```python
from build123d import *

# Parameters (mm, degrees)
SKETCH1_R          = 27.5
SKETCH1_R_2        = 48.5
BASE_EXTRUDE_DEPTH = 10


with BuildPart() as part:
    # Sketch1 → Base-Extrude (new body)
    with BuildSketch(Plane.XY):
        with BuildLine():
            Line((70.930675146, 17.258022001), (31.072409725, 181.075965699))
            ThreePointArc((31.072409725, 181.075965699), (-37.180312094, 232.965036888), (-101.966927205, 176.808076081))
            Line((-101.966927205, 176.808076081), (-104.698317648, 161.317591117))
            ThreePointArc((-104.698317648, 161.317591117), (-124.339394775, 129.702595413), (-160.381803445, 120.416872968))
            ThreePointArc((-160.381803445, 120.416872968), (-227.936557036, 127.643740719), (-295.749262378, 131.804190759))
            ThreePointArc((-295.749262378, 131.804190759), (-329.964920671, 135.496946415), (-363.349263399, 143.853583144))
            Line((-363.349263399, 143.853583144), (-458.454915028, 174.755282581))
            ThreePointArc((-458.454915028, 174.755282581), (-464.263200822, 172.612492824), (-463.535533906, 166.464466094))
            Line((-463.535533906, 166.464466094), (-422.516106966, 125.445039154))
            ThreePointArc((-422.516106966, 125.445039154), (-372.592477248, 89.023301508), (-313.933303895, 69.580741007))
            ThreePointArc((-313.933303895, 69.580741007), (-204.337272048, 38.490168586), (-104.328864588, -16.064687542))
            Line((-104.328864588, -16.064687542), (-41.871079854, -59.798099233))
            ThreePointArc((-41.871079854, -59.798099233), (41.176771055, -60.278300619), (70.930675146, 17.258022001))
        make_face()
        Circle(SKETCH1_R, mode=Mode.SUBTRACT)
        with Locations((-35, 165)):
            Circle(SKETCH1_R_2, mode=Mode.SUBTRACT)
    extrude(amount=BASE_EXTRUDE_DEPTH)


solid = part.part
```
Could you check a few things on this model? Use its own coordinates, in mm. A direction names the side the tool comes from. Coordinates: 2 decimals unless noted, no trailing zeros. Write each loop counter-clockwise with the first axis right and the second up, starting at its lowest first coordinate (ties: lowest second). Pieces come first, ordered by that corner, then holes. Notation, with made-up numbers: (-26, -28) - (7, -28) arc R15 cw to (7, -15) - close; hole circle Ø10 at (8.5, 60.5). An arc over 180 degrees is marked (long way). Use a Markdown table: item, result.
Q1. Imagine slicing it at B-B (z = 1.75). List the corners of the cut face in (x, y) for me, and give its area (3 significant figures).
Geometry check:
| item | result |
|---|---|
| outline | (-463.54, 166.46) - (-422.52, 125.45) arc R200 ccw to (-313.93, 69.58) arc R512 cw to (-104.33, -16.06) - (-41.87, -59.8) arc R73 ccw to (70.93, 17.26) - (31.07, 181.08) arc R68 ccw to (-101.97, 176.81) - (-104.7, 161.32) arc R50 cw to (-160.38, 120.42) arc R1500 ccw to (-295.75, 131.8) arc R250 cw to (-363.35, 143.85) - (-458.45, 174.76) arc R5 ccw to start; hole circle Ø97 at (-35, 165); hole circle Ø55 at (0, 0) |
| area | 59,600 mm2 |
Q2. Imagine slicing it at D-D (y = 138.5). List the corners of the cut face in (x, z) for me.
Geometry check:
| item | result |
|---|---|
| outline | (-435.57, 0) - (-344.35, 0) - (-344.35, 10) - (-435.57, 10) - close; (-115.11, 0) - (-75.62, 0) - (-75.62, 10) - (-115.11, 10) - close; (5.62, 0) - (41.43, 0) - (41.43, 10) - (5.62, 10) - close |
Q3. I'm going to push flat-ended pins straight in: pin 1 Ø1 at (x, z) = (-78, 5) entering from +Y; pin 2 Ø1.5 at (x, z) = (-313, 3) entering from -Y; pin 3 Ø6 at (y, z) = (-32.5, 9) entering from -X. Where does each tip first touch, or does it pass through?
Geometry check:
| item | result |
|---|---|
| pin 1 | stops at y = 218.08 |
| pin 2 | stops at y = 69.3 |
| pin 3 | stops at x = -85.14 |
Q4. Imagine slicing it at A-A (y = 8). List the corners of the cut face in (x, z) for me.
Geometry check:
| item | result |
|---|---|
| outline | (-142.11, 0) - (-26.31, 0) - (-26.31, 10) - (-142.11, 10) - close; (26.31, 0) - (72.56, 0) - (72.56, 10) - (26.31, 10) - close |
Q5. Imagine slicing it at C-C (x = -35). List the corners of the cut face in (y, z) for me, and give its area (3 significant figures).
Geometry check:
| item | result |
|---|---|
| outline | (-64.06, 0) - (116.5, 0) - (116.5, 10) - (-64.06, 10) - close; (213.5, 0) - (233, 0) - (233, 10) - (213.5, 10) - close |
| area | 2,000 mm2 |
Q6. Thinking about a two-plate mould opening in Y: for faces 1 (the flat face through (-103.314, 169.171, 4.93)), 2 (the cylindrical face through (-5.961, -26.846, 4.93)), 3 (the flat face through (-73.537, -37.625, 4.93)), 4 (the flat face through (-140, 82, 0)), which applies, +Y half, -Y half, draft (parallel to the pull), parting line (faces both ways), or undercut?
Geometry check:
| item | result |
|---|---|
| face 1 | +Y half |
| face 2 | undercut |
| face 3 | -Y half |
| face 4 | draft |
Q7. Which directions (+Z, -Z, +X, -X, +Y, -Y) give clear straight access to the entire face, cutting with the end or side of a thin tool? Please do faces 5 (the cylindrical face through (-45.514, 117.653, 4.93)), 6 (the cylindrical face through (-226.989, 127.564, 4.93)).
Geometry check:
| item | result |
|---|---|
| face 5 | +Z, -Z |
| face 6 | +Z, -Z, +Y |
Q8. Please list where these lines run through material, in increasing order: L1, parallel to Y at x = 0, z = 6; L2, parallel to Y at x = 1, z = 9.25; L3, parallel to X at y = -18, z = 1.
Geometry check:
| item | result |
|---|---|
| L1 | y = -73 to -27.5, 27.5 to 131.43, 198.57 to 223.3 |
| L2 | y = -72.99 to -27.48, 27.48 to 132.5, 197.5 to 222.69 |
| L3 | x = -101.56 to -20.79, 20.79 to 70.75 |
